For this review, take the finished solid that the model builds, in its own axes (mm). A direction names the side the tool comes from. Give positions to 0.01 mm unless a question says otherwise; leave off trailing zeros. Loops run counter-clockwise (first coordinate to the right, second up) from the corner with the lowest first, then second, coordinate; pieces in that order, holes last. Notation, with made-up numbers: (73, 27) - (86, 27) arc R18 cw to (86, 44) - close; hole circle Ø5 at (78.25, -33.5). An arc over 180 degrees is marked (long way). Put each result on its own line as item: value.
from build123d import *

# Parameters (mm, degrees)
SKETCH1_R           = 2.5
BOSS_EXTRUDE1_DEPTH = 3
SKETCH2_W           = 20
SKETCH2_H           = 45.01020326
SKETCH2_R           = 2.75
BOSS_EXTRUDE2_DEPTH = 3
BOSS_EXTRUDE3_DEPTH = 3


with BuildPart() as part:
    # Sketch1 → Boss-Extrude1 (new body)
    with BuildSketch(Plane.XY):
        Polygon((0, 0), (0.958330597, 45), (27, 45), (27, 0), align=None)
        with Locations((17.5, 36)):
            Circle(SKETCH1_R, mode=Mode.SUBTRACT)
        with Locations((17.5, 9)):
            Circle(SKETCH1_R, mode=Mode.SUBTRACT)
        with Locations((9.5, 22.5)):
            Circle(SKETCH1_R, mode=Mode.SUBTRACT)
    extrude(amount=BOSS_EXTRUDE1_DEPTH)

    # Sketch2 → Boss-Extrude2 (add)
    with BuildSketch(Plane(origin=(0, 0, 0), x_dir=(0, 0, 1), z_dir=(-0.999773312, 0.021291408, 0))):
        with Locations((10, 22.50510163)):
            Rectangle(SKETCH2_W, SKETCH2_H)
        with Locations((10, 36.01020326)):
            Circle(SKETCH2_R, mode=Mode.SUBTRACT)
        with Locations((10, 9)):
            Circle(SKETCH2_R, mode=Mode.SUBTRACT)
    extrude(amount=BOSS_EXTRUDE2_DEPTH)

    # Sketch3 → Boss-Extrude3 (add)
    with BuildSketch(Plane(origin=(0.958330597, 45, 0), x_dir=(0.999773312, -0.021291408, 0), z_dir=(0.021291408, 0.999773312, 0))):
        Polygon((0, -20), (26.035766076, -3), (26.035766076, 0), (-3, 0), (-3, -20), align=None)
    extrude(amount=BOSS_EXTRUDE3_DEPTH)


solid = part.part
1) Take a section at A-A on x = 17.5. State the section outline as (y, z) points, and give its area (3 significant figures).
Geometry check:
outline: (0, 0) - (6.5, 0) - (6.5, 3) - (0, 3) - close; (11.5, 0) - (33.5, 0) - (33.5, 3) - (11.5, 3) - close; (38.5, 0) - (47.65, 0) - (47.65, 9.24) - (44.65, 9.2) - (44.65, 3) - (38.5, 3) - close
area: 132 mm²
2) Take a section at D-D on x = 9.5. State the section outline as (y, z) points.
Geometry check:
outline: (0, 0) - (20, 0) - (20, 3) - (0, 3) - close; (25, 0) - (47.82, 0) - (47.82, 14.46) - (44.82, 14.42) - (44.82, 3) - (25, 3) - close
3) For faces 4 (the face through (27, 23, 1)), 5 (the face through (-0.764, 33.594, 11.269)), 6 (the face through (13, 23, 0)), list the 3-axis set-ups (+Z, -Z, +X, -X, +Y, -Y) from which the entire face can be reached by the end or side of a thin tool; tool diameter is ignored.
Geometry check:
face 4: +Z, -Z, +X, -Y
face 5: none
face 6: -Z, +X, -X, +Y, -Y
4) Wall thickness on line 1 (Y direction, x = 17.5, z = 0.95); line 2 (Z direction, x = 17.5, y = 18); line 3 (Z direction, x = -0.5, y = 38.5): over which ranges is each line inside the solid? List them lowest first.
Geometry check:
line 1: y = 0 to 6.5, 11.5 to 33.5, 38.5 to 47.65
line 2: z = 0 to 3
line 3: z = 0 to 8.79, 11.21 to 20
5) Take a section at B-B on y = 22. State the section outline as (x, z) points, and give its area (3 significant figures).
Geometry check:
outline: (-2.53, 0) - (7.05, 0) - (7.05, 3) - (0.47, 3) - (0.47, 20) - (-2.53, 20) - close; (11.95, 0) - (27, 0) - (27, 3) - (11.95, 3) - close
area: 125 mm²
6) Take a section at C-C on z = 2. State the section outline as (x, y) points, and give its area (3 significant figures).
Geometry check:
outline: (-3, 0.06) - (0, 0) - (27, 0) - (27, 45) - (27.05, 47.44) - (-1.98, 48.06) - close; hole circle Ø5 at (9.5, 22.5); hole circle Ø5 at (17.5, 9); hole circle Ø5 at (17.5, 36)
area: 1,350 mm²
7) Insertion check: pin 1 Ø8 at (x, y) = (17.5, 9) entering from +Z; pin 2 Ø1.5 at (y, z) = (5, 13.5) entering from +X; pin 3 Ø10 at (y, z) = (38.5, 17.5) entering from +X. Each pin has a flat end and moves straight along its axis. Give the tip position at first contact, or say it passes through.
Geometry check:
pin 1: stops at z = 3
pin 2: stops at x = 0.12
pin 3: stops at x = 0.93
8) Draft analysis for pull direction Y (two halves, no side actions). For faces 1 (the face through (-1, 24, 20)), 2 (the face through (-1.27, 9.86, 12.62)), 3 (the face through (14, 0, 1)), state which applies: pulls with the +Y half, pulls with the -Y half, needs draft (parallel to the pull), parting line crosses it, or undercut.
Geometry check:
face 1: needs draft
face 2: undercut
face 3: pulls with the -Y half
